CAD build for the part. Positions are in the model's coordinates, mm. Face numbers are marked on the shaded views. A direction names the side the tool comes from. Coordinates: 2 decimals unless noted, no trailing zeros. Loops run counter-clockwise (first coordinate to the right, second up) from the corner with the lowest first, then second, coordinate; pieces in that order, holes last. Notation, with made-up numbers: (74, -22.5) -> (90, -22.5) arc R18 ccw to (90, -0.5) -> close; hole circle Ø1 at (2, 49.25). An arc over 180 degrees is marked (long way). Write each question's results on one line, items separated by ' | '.
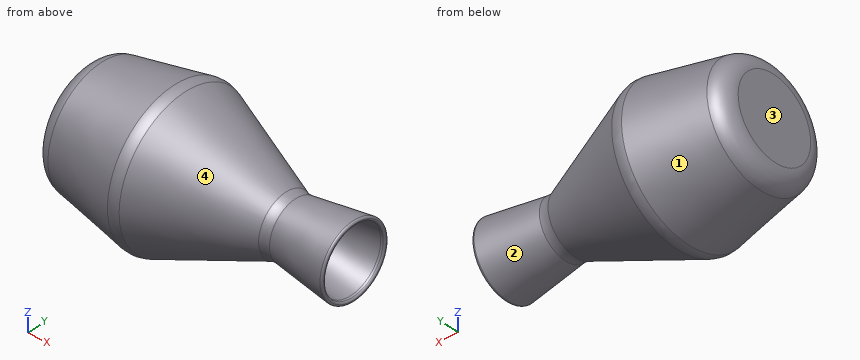
from build123d import *

# Parameters (mm, degrees)
FILLET_1_R = 1
FILLET_4_R = 10


with BuildPart() as part:
    # 스케치2 → 회전5 (revolve)
    with BuildSketch(Plane(origin=(0, 0, 0), x_dir=(1, 0, 0), z_dir=(0, 1, 0)), mode=Mode.PRIVATE) as revolve_5_sk:
        Polygon((-78.828533155, 4.583054253), (-78.828533155, 34.583054253), (-28.828533155, 44.583054253), (31.171466845, 19.583054253), (66.171466845, 24.583054253), (66.171466845, 22.562749164), (64.171466845, 22.277034878), (30.909884451, 17.525380251), (-29.034574551, 42.502238168), (-76.828533155, 32.943446448), (-76.828533155, 4.583054253), align=None)
    revolve(revolve_5_sk.sketch.rotate(Axis((-92.184862693, 0, -4.583054253), (1, 0, 0)), 180), axis=Axis((-92.184862693, 0, -4.583054253), (1, 0, 0)))

    # 필렛1
    fillet_1_edges = [part.edges().sort_by_distance(p)[0] for p in [
        (66.171466845, 0, -22.562749164),
        (66.171466845, 0, -24.583054253),
    ]]
    fillet(fillet_1_edges, radius=FILLET_1_R - 0.0001)  # a hair under: the kernel refuses the full size

    # 필렛4
    fillet_4_edges = [part.edges().sort_by_distance(p)[0] for p in [
        (-76.828533155, 0, -32.943446448),
        (-29.034574551, 0, -42.502238168),
        (30.909884451, 0, -17.525380251),
        (31.171466845, 0, -19.583054253),
        (-28.828533155, 0, -44.583054253),
        (-78.828533155, 0, -34.583054253),
    ]]
    fillet(fillet_4_edges, radius=FILLET_4_R)


solid = part.part
1) Which spindle directions (+Z, -Z, +X, -X, +Y, -Y) get a long thin tool onto all of the face, cutting with end or side? Do the marked faces 3 and 4. Say none if no direction does.
Outcome:
face 3: +Z, -Z, -X, +Y, -Y | face 4: none
2) Drill centre lines: L1, parallel to Z at x = -54, y = 18.5; L2, parallel to Y at x = -31, z = -31.5; L3, parallel to X at y = 20, z = -18. Where is each one in solid material? Low to high. Write a range as from..to.
Outcome:
L1: z = -34.25..-31.82, 22.65..25.09 | L2: y = -28.95..-26.07, 26.07..28.95 | L3: x = -78.56..-76.03, 4.17..9.37
3) Slice it at A-A (x = -11.5). Write the cut outline in (y, z).
Outcome:
outline: circle Ø65.56 at (0, -4.58); hole circle Ø61.23 at (0, -4.58)
4) Two-plate mould, pull along X, no slides. Class the marked faces 1 and 2: pulls with the +X half, pulls with the -X half, needs draft (parallel to the pull), parting line crosses it, or undercut.
Outcome:
face 1: pulls with the -X half | face 2: undercut
5) Slice it at B-B (x = 4.5). Write the cut outline in (y, z).
Outcome:
outline: circle Ø52.23 at (0, -4.58); hole circle Ø47.89 at (0, -4.58)
6) Pin check, flat tips, straight feed: pin 1 (6 mm diameter, centred on y = -25, z = -14, fed in from -X); pin 2 (6 mm diameter, centred on x = -9.5, z = -31, fed in from +Y); pin 3 (2 mm diameter, centred on x = -45, y = -28.5, fed in from +Z). Stop position of each tip, or through.
Outcome:
pin 1: stops at x = -78.64 | pin 2: stops at y = 22.22 | pin 3: stops at z = 19.86
